```python
from build123d import *

# Parameters (mm, degrees)
BOSS_EXTRUDE1_DEPTH      = 120
SKETCH1_3_W              = 80
SKETCH1_3_H              = 120
BOSS_EXTRUDE2_DEPTH      = 80
BOSS_EXTRUDE3_DEPTH      = 120
SKETCH1_5_W              = 80
SKETCH1_5_H              = 120
BOSS_EXTRUDE4_DEPTH      = 120
SKETCH2_W                = 80
SKETCH2_H                = 40
BOSS_EXTRUDE5_DEPTH      = 160
SKETCH2_8_W              = 80
SKETCH2_8_H              = 40
BOSS_EXTRUDE6_DEPTH      = 80
SKETCH2_9_W              = 80
SKETCH2_9_H              = 40
BOSS_EXTRUDE7_DEPTH      = 160
CUT_EXTRUDE20_DEPTH      = 224.60679775
CUT_EXTRUDE20_DEPTH_BACK = 121


with BuildPart() as part:
    # Sketch1 → Boss-Extrude1 (new body)
    with BuildSketch(Plane.XY):
        Polygon((120, -100), (120, -20), (40, -20), (-120, -20), (-120, -100), align=None)
    extrude(amount=BOSS_EXTRUDE1_DEPTH)

    # Sketch1<3> → Boss-Extrude2 (add)
    with BuildSketch(Plane.XY):
        with Locations((80, 40)):
            Rectangle(SKETCH1_3_W, SKETCH1_3_H)
    extrude(amount=BOSS_EXTRUDE2_DEPTH)

    # Sketch1<4> → Boss-Extrude3 (add)
    with BuildSketch(Plane.XY):
        Polygon((120, -100), (120, -20), (40, -20), (-120, -20), (-120, -100), align=None)
    extrude(amount=-BOSS_EXTRUDE3_DEPTH)

    # Sketch1<5> → Boss-Extrude4 (add)
    with BuildSketch(Plane.XY):
        with Locations((80, 40)):
            Rectangle(SKETCH1_5_W, SKETCH1_5_H)
    extrude(amount=-BOSS_EXTRUDE4_DEPTH)

    # Sketch2 → Boss-Extrude5 (add)
    with BuildSketch(Plane.ZY.offset(-40)):
        with Locations((-80, 0)):
            Rectangle(SKETCH2_W, SKETCH2_H)
    extrude(amount=BOSS_EXTRUDE5_DEPTH)

    # Sketch2<8> → Boss-Extrude6 (add)
    with BuildSketch(Plane.ZY.offset(-40)):
        with Locations((-80, 80)):
            Rectangle(SKETCH2_8_W, SKETCH2_8_H)
    extrude(amount=BOSS_EXTRUDE6_DEPTH)

    # Sketch2<9> → Boss-Extrude7 (add)
    with BuildSketch(Plane.ZY.offset(-40)):
        with Locations((-80, 40)):
            Rectangle(SKETCH2_9_W, SKETCH2_9_H)
    extrude(amount=BOSS_EXTRUDE7_DEPTH)

    # Sketch4 → Cut-Extrude20 (cut, two sides: drawn at the far end of the back side and taken through both)
    with BuildSketch(Plane.XY.offset(-40).offset(-CUT_EXTRUDE20_DEPTH_BACK)):
        Polygon((-120, 20), (-40, 60), (-120, 60), align=None)
    extrude(amount=CUT_EXTRUDE20_DEPTH + CUT_EXTRUDE20_DEPTH_BACK, mode=Mode.SUBTRACT)


solid = part.part
```
Geometry check sheet. Reference: the model listing, model coordinates, mm. A direction names the side the tool comes from. Round coordinates to 2 decimals unless told otherwise and drop trailing zeros. Loops run counter-clockwise (first coordinate to the right, second up) from the corner with the lowest first, then second, coordinate; pieces in that order, holes last. Notation, with made-up numbers: M -4.75,-5.5 L 14.25,-5.5 A16 cw 14.25,13.5 Z; hole C 79,20.25 d1. An arc over 180 degrees is marked long. Return JSON: item names as keys, results as strings. Group by question number.
(1) Section check A-A, the plane y = 69.5. Enter the section's corners in (x, z), and give its area (3 significant figures).
(2) Scan lines: line 1 along Z through (x, y) = (-29, 69); line 2 along X through (y, z) = (16, 71.5); line 3 along Z through (x, y) = (95.5, 15). Record each from-to range of solid material in increasing order. Write a range as [from, to].
(3) Section check B-B, the plane x = -100. Enter the section's corners in (y, z).
(4) Go/stop test with flat-tipped pins: pin 1 (1.5 mm diameter, centred on x = -31, z = -39, fed in from +Y); pin 2 (24 mm diameter, centred on x = 62.5, y = 61.5, fed in from +Z); pin 3 (3 mm diameter, centred on y = 44, z = 78, fed in from -X); pin 4 (8 mm diameter, centred on y = 28, z = 83.5, fed in from +X). Record where each tip stops, or that it passes through.
(5) Set-up check for faces 1 (the face through (79, 41, 80)), 2 (the face through (-21, 26, -40)), 3 (the face through (-40, 80, -81)): record each of +Z, -Z, +X, -X, +Y, -Y from which the full face is reachable in a straight line by a thin tool's end or side.
Data:
{
 "1": {"outline": "M -40,-120 L 120,-120 L 120,80 L 40,80 L 40,-40 L -40,-40 Z", "area": "22,400 mm²"},
 "2": {"line 1": "[-120, -40]", "line 2": "[40, 120]", "line 3": "[-120, 80]"},
 "3": {"outline": "M -100,-120 L 30,-120 L 30,-40 L -20,-40 L -20,120 L -100,120 Z"},
 "4": {"pin 1": "y = -20", "pin 2": "z = 80", "pin 3": "x = 40", "pin 4": "x = 120"},
 "5": {"face 1": "+Z, +X, -X, +Y", "face 2": "+Z, -X, +Y", "face 3": "+Z, -Z, -X, +Y"}
}
